Part model, mm, in its own coordinate system. A direction names the side the tool comes from. Give positions to 0.01 mm unless a question says otherwise; leave off trailing zeros. Write each loop counter-clockwise with the first axis right and the second up, starting at its lowest first coordinate (ties: lowest second). Pieces come first, ordered by that corner, then holes. Notation, with made-up numbers: M 5.25,55 L 64.25,55 A15 cw 64.25,71 Z; hole C 21.5,85 d9. An arc over 180 degrees is marked long. Use CSV: the item, a comma, the result in double quotes. Start each with the question number.
1. Mould opens along X. For faces 1 (the face through (0, 0, -122)), 2 (the face through (1, 0, 122)), 3 (the face through (-136.152, 0, -123)) say: pulls with the +X half, pulls with the -X half, needs draft (parallel to the pull), parting line crosses it, or undercut.
2. 3-axis set-ups, long thin cutter, end or side, ignore diameter. For faces 4 (the face through (86, 0, -133)), 5 (the face through (91, 0, 43)), 6 (the face through (112.106, -0.071, -78.879)), 7 (the face through (-91, 0, 45)), 8 (the face through (9, 5.05, -118)): which of +Z, -Z, +X, -X, +Y, -Y reach the whole face in a straight line?
3. Band-saw the part on C-C, the plane y = 2.75. Count the separate pieces of the cut face and the enclosed holes in it, then the cut area to 3 significant figures.
4. Band-saw the part on B-B, the plane x = 63.5. List the corners of the cut face in (y, z).
5. Drill centre lines: line 1 along X through (y, z) = (-0.25, 66); line 2 along Z through (x, y) = (-77.5, 3.5); line 3 along X through (y, z) = (0, -108). Where is each one in solid material? Low to high. Write a range as from..to.
6. Drop flat-ended pins along their axis: pin 1 Ø2.5 at (x, y) = (105.5, 1.5) entering from +Z; pin 2 Ø5 at (y, z) = (-1.5, -79) entering from +X; pin 3 Ø3 at (y, z) = (-2, 45) entering from -X. Give the stop position or say it passes through.
7. Band-saw the part on A-A, the plane z = 75.5. List the corners of the cut face in (x, y).
from build123d import *

# Parameters (mm, degrees)
F0_W     = 164
F0_H     = 226
F1_DEPTH = 5.05
F2_R     = 5
F3_R     = 5


with BuildPart() as f1:
    # F0 (on Front) → F1 (new body, symmetric)
    with BuildSketch(Plane.XZ):
        with BuildLine():
            ThreePointArc((-136.1519984865, -128), (-134.6875323924, -131.5355339059), (-131.1519984865, -133))
            Line((-131.1519984865, -133), (-41.1519984865, -133))
            ThreePointArc((-41.1519984865, -133), (-38.493646634, -132.2347568323), (-36.6490090186, -130.1732661714))
            Line((-36.6490090186, -130.1732661714), (-34.0686259291, -124.8267338286))
            ThreePointArc((-34.0686259291, -124.8267338286), (-32.2239883137, -122.7652431677), (-29.5656364612, -122))
            Line((-29.5656364612, -122), (29.5656364612, -122))
            ThreePointArc((29.5656364612, -122), (32.2239883137, -122.7652431677), (34.0686259291, -124.8267338286))
            Line((34.0686259291, -124.8267338286), (36.6490090186, -130.1732661714))
            ThreePointArc((36.6490090186, -130.1732661714), (38.493646634, -132.2347568323), (41.1519984865, -133))
            Line((41.1519984865, -133), (131.1519984865, -133))
            ThreePointArc((131.1519984865, -133), (134.6875323924, -131.5355339059), (136.1519984865, -128))
            Line((136.1519984865, -128), (136.1519984865, -118.9447689056))
            ThreePointArc((136.1519984865, -118.9447689056), (134.6875323924, -115.4092349997), (131.1519984865, -113.9447689056))
            Line((131.1519984865, -113.9447689056), (127.0574602485, -113.9447689056))
            ThreePointArc((127.0574602485, -113.9447689056), (123.5219263425, -112.4803028116), (122.0574602485, -108.9447689056))
            add(Edge.make_bspline(
                [(122.0574602485, -108.9447689056), (123.931935402, -85.3492312011), (127.0202597137, -46.4739905223), (106.0084033701, -39.5765251934), (97.7498069406, -36.8655137718)],
                knots=[0, 0, 0, 0, 0.6069554115, 1, 1, 1, 1], degree=3))
            Line((97.7498069406, -36.8655137718), (94.2721525095, -36.8655137718))
            ThreePointArc((94.2721525095, -36.8655137718), (91.958391281, -35.9071224908), (91, -33.5933612622))
            Line((91, -33.5933612622), (91, 122))
            Line((91, 122), (-91, 122))
            Line((-91, 122), (-91, -33.5933612622))
            ThreePointArc((-91, -33.5933612622), (-91.958391281, -35.9071224908), (-94.2721525095, -36.8655137718))
            Line((-94.2721525095, -36.8655137718), (-97.7498069406, -36.8655137718))
            add(Edge.make_bspline(
                [(-122.0574602485, -108.9447689056), (-123.931935402, -85.3492312011), (-127.0202597137, -46.4739905223), (-106.0084033701, -39.5765251934), (-97.7498069406, -36.8655137718)],
                knots=[0, 0, 0, 0, 0.6069554115, 1, 1, 1, 1], degree=3))
            ThreePointArc((-122.0574602485, -108.9447689056), (-123.5219263425, -112.4803028116), (-127.0574602485, -113.9447689056))
            Line((-127.0574602485, -113.9447689056), (-131.1519984865, -113.9447689056))
            ThreePointArc((-131.1519984865, -113.9447689056), (-134.6875323924, -115.4092349997), (-136.1519984865, -118.9447689056))
            Line((-136.1519984865, -118.9447689056), (-136.1519984865, -128))
        make_face()
        with BuildLine():
            Line((-112.9490544478, -100.6573063768), (-111.2859340244, -57.7014318636))
            ThreePointArc((-111.2859340244, -57.7014318636), (-109.7561453304, -54.291595458), (-106.2896773219, -52.8948716819))
            Line((-106.2896773219, -52.8948716819), (-101.2297698661, -52.8948716819))
            ThreePointArc((-101.2297698661, -52.8948716819), (-97.6942359602, -54.359337776), (-96.2297698661, -57.8948716819))
            Line((-96.2297698661, -57.8948716819), (-96.2297698661, -100.8894341588))
            ThreePointArc((-96.2297698661, -100.8894341588), (-97.987129179, -105.1320748459), (-102.2297698661, -106.8894341588))
            Line((-102.2297698661, -106.8894341588), (-106.9535464048, -106.8894341588))
            ThreePointArc((-106.9535464048, -106.8894341588), (-111.2774778735, -105.049195769), (-112.9490544478, -100.6573063768))
        make_face(mode=Mode.SUBTRACT)
        with BuildLine():
            Line((96.2297698661, -100.8894341588), (96.2297698661, -57.8948716819))
            ThreePointArc((96.2297698661, -57.8948716819), (97.6942359602, -54.359337776), (101.2297698661, -52.8948716819))
            Line((101.2297698661, -52.8948716819), (106.2896773219, -52.8948716819))
            ThreePointArc((106.2896773219, -52.8948716819), (109.7561453304, -54.291595458), (111.2859340244, -57.7014318636))
            Line((111.2859340244, -57.7014318636), (112.9490544478, -100.6573063768))
            ThreePointArc((112.9490544478, -100.6573063768), (111.2774778735, -105.049195769), (106.9535464048, -106.8894341588))
            Line((106.9535464048, -106.8894341588), (102.2297698661, -106.8894341588))
            ThreePointArc((102.2297698661, -106.8894341588), (97.987129179, -105.1320748459), (96.2297698661, -100.8894341588))
        make_face(mode=Mode.SUBTRACT)
        Rectangle(F0_W, F0_H, mode=Mode.SUBTRACT)
    extrude(amount=F1_DEPTH, both=True)

    # F2
    f2_edges = [f1.edges().sort_by_distance(p)[0] for p in [
        (97.749807, 2.525, -36.865514),
        (97.749807, -2.525, -36.865514),
    ]]
    fillet(f2_edges, radius=F2_R)

    # F3
    f3_edges = [f1.edges().sort_by_distance(p)[0] for p in [
        (-97.749807, 2.525, -36.865514),
        (-97.749807, -2.525, -36.865514),
    ]]
    fillet(f3_edges, radius=F3_R)


solid = f1.part
Output:
1,face 1,"undercut"
1,face 2,"needs draft"
1,face 3,"pulls with the -X half"
2,face 4,"-Z, +X, -X, +Y, -Y"
2,face 5,"+Z, +X, +Y, -Y"
2,face 6,"+Y, -Y"
2,face 7,"+Z, -X, +Y, -Y"
2,face 8,"+Z, -Z, +X, -X, +Y"
3,separate pieces,"1"
3,enclosed holes,"3"
3,area,"13,200 mm²"
4,outline,"M -5.05,-133 L 5.05,-133 L 5.05,-113 L -5.05,-113 Z; M -5.05,113 L 5.05,113 L 5.05,122 L -5.05,122 Z"
5,line 1,"x = -91..-82, 82..91"
5,line 2,"z = -133..-113, 113..122"
5,line 3,"x = -122.13..-82, 82..122.13"
6,pin 1,"stops at z = -39.11"
6,pin 2,"stops at x = 123.78"
6,pin 3,"stops at x = -91"
7,outline,"M -91,-5.05 L -82,-5.05 L -82,5.05 L -91,5.05 Z; M 82,-5.05 L 91,-5.05 L 91,5.05 L 82,5.05 Z"
